Check sheet for the modelled part. Datum: model origin and axes. Units: mm. A direction names the side the tool comes from. Round coordinates to 2 decimals unless told otherwise and drop trailing zeros. Write each loop counter-clockwise with the first axis right and the second up, starting at its lowest first coordinate (ties: lowest second). Pieces come first, ordered by that corner, then holes. Notation, with made-up numbers: (-5.75, 61) - (51.25, 61) arc R22 ccw to (51.25, 71) - close; hole circle Ø11 at (-40, 51). An arc over 180 degrees is marked (long way). Answer as a JSON object with one key per item and string values. Group by question number.
Item 1: Gauge pin test, flat ends, axial feed: P1, Ø8, axis at x = -26.4, y = -15.24, coming from the -Z side; P2, Ø1, axis at y = -29.5, z = 25.5, coming from the +X side; P3, Ø1.5, axis at x = 28, z = 24, coming from the -Y side; P4, Ø3, axis at y = 35, z = 4.5, coming from the -X side. Record the tip position at first contact, or that the pin passes through.
Item 2: Thickness scan on line 1 (Y direction, x = 0, z = 5); line 2 (X direction, y = -11, z = 7.5); line 3 (X direction, y = 13, z = 17.5). Record the ranges inside material, lowest first.
Item 3: Release check for a two-part mould opening along X. For faces 3 (the flat face through (11, 1, 0)), 4 (the cylindrical face through (-27.058, -10.203, 12.878)), 5 (the cylindrical face through (-6.944, -52.886, 17.531)) record: pulls with the +X half, pulls with the -X half, needs draft (parallel to the pull), parting line crosses it, or undercut.
Item 4: Sectioned sample at C-C on z = 10.5. Record the boundary of the cut face in (x, y), plus the area to 3 significant figures.
Item 5: Set-up check for faces 1 (the flat face through (-36, 13, 35.56)), 2 (the flat face through (-1, -8, 25.4)): record each of +Z, -Z, +X, -X, +Y, -Y from which the full face is reachable in a straight line by a thin tool's end or side.
Item 6: Sectioned sample at B-B on y = 0. Record the boundary of the cut face in (x, z).
Item 7: Sectioned sample at D-D on y = 15.24. Record the boundary of the cut face in (x, z), plus the area to 3 significant figures.
Item 8: Sectioned sample at A-A on x = 0. Record the boundary of the cut face in (y, z).
Autodesk Inventor part; units mm, degrees
ref_plane "YZ Plane" through (0, 0, 0) normal (1, 0, 0) x (0, 1, 0)
ref_plane "XZ Plane" through (0, 0, 0) normal (0, 1, 0) x (-1, 0, 0)
ref_plane "XY Plane" through (0, 0, 0) normal (0, 0, 1) x (1, 0, 0)
sketch "Sketch1" plane through (0, 0, 0) normal (0, 0, 1) x (1, 0, 0)
  circle A0 centre (0, 0) radius 53.34
  dimension "d0" = 106.68
extrude "Extrusion1" add sketch "Sketch1" along normal blind 35.56
sketch "Sketch2" plane through (0, 0, 35.56) normal (0, 0, 1) x (1, 0, 0)
  circle A0 centre (0, 0) radius 38.1
  dimension "d3" = 76.2
extrude "Extrusion2" cut sketch "Sketch2" against normal blind 10.16
sketch "Sketch3" plane through (0, 0, 25.4) normal (0, 0, 1) x (1, 0, 0)
  line L0 (-74.676, 0) -> (74.676, 0) construction
  line L1 (0, -74.676) -> (0, 74.676) construction
  circle A0 centre (0, 0) radius 30.48
  circle A1 centre (0, 30.48) radius 5.08
  circle A2 centre (-26.3965, 15.24) radius 5.08
  circle A3 centre (-26.3965, -15.24) radius 5.08
  circle A4 centre (0, -30.48) radius 5.08
  circle A5 centre (26.3965, -15.24) radius 5.08
  circle A6 centre (26.3965, 15.24) radius 5.08
  circle A7 centre (0, 0) radius 5.08
  dimension "d6" = 60.96
  dimension "d7" = 10.16
  dimension "d10" = 360
  dimension "d14" = 10.16
extrude "Extrusion3" cut sketch "Sketch3" against normal through all contours A6 A0 | A0 A6 | A5 A0 | A0 A5 | A1 A0 | A0 A1 | A4 A0 | A0 A4 | A2 A0 | A0 A2 | A3 A0 | A0 A3 | A7
sketch "Sketch4" plane through (0, 0, 0) normal (1, 0, 0) x (0, 1, 0)
  line L0 (-38.1, 25.4) -> (38.1, 25.4)
  line L1 (53.34, 35.56) -> (-53.34, 35.56)
  line L2 (53.34, 0) -> (-53.34, 0)
  line L3 (-5.08, 25.4) -> (-5.08, 0)
  line L4 (-5.08, 0) -> (-25.4, 0)
  line L5 (-25.4, 0) -> (-25.4, 25.4)
  line L6 (-25.4, 25.4) -> (-5.08, 25.4)
  line L7 (5.08, 0) -> (5.08, 25.4)
  line L8 (5.08, 25.4) -> (25.4, 25.4)
  line L9 (25.4, 25.4) -> (25.4, 0)
  line L10 (25.4, 0) -> (5.08, 0)
  line L11 (53.34, 35.56) -> (53.34, 0)
  line L12 (53.34, 0) -> (35.56, 0)
  line L13 (35.56, 0) -> (35.56, 25.4)
  line L14 (35.56, 25.4) -> (38.1, 25.4)
  line L15 (38.1, 25.4) -> (38.1, 35.56)
  line L16 (38.1, 35.56) -> (53.34, 35.56)
  line L17 (-53.34, 0) -> (-53.34, 35.56)
  line L18 (-53.34, 35.56) -> (-38.1, 35.56)
  line L19 (-38.1, 35.56) -> (-38.1, 25.4)
  line L20 (-38.1, 25.4) -> (-35.56, 25.4)
  line L21 (-35.56, 25.4) -> (-35.56, 0)
  line L22 (-35.56, 0) -> (-53.34, 0)
  line L23 (-5.08, 25.4) -> (-5.08, 0)
  line L24 (-5.08, 0) -> (-25.4, 0)
  line L25 (-25.4, 0) -> (-25.4, 25.4)
  line L26 (-25.4, 25.4) -> (-5.08, 25.4)
  line L27 (5.08, 0) -> (5.08, 25.4)
  line L28 (5.08, 25.4) -> (25.4, 25.4)
  line L29 (25.4, 25.4) -> (25.4, 0)
  line L30 (25.4, 0) -> (5.08, 0)
  line L31 (53.34, 35.56) -> (53.34, 0)
  line L32 (53.34, 0) -> (35.56, 0)
  line L33 (35.56, 0) -> (35.56, 25.4)
  line L34 (35.56, 25.4) -> (38.1, 25.4)
  line L35 (38.1, 25.4) -> (38.1, 35.56)
  line L36 (38.1, 35.56) -> (53.34, 35.56)
  line L37 (-53.34, 0) -> (-53.34, 35.56)
  line L38 (-53.34, 35.56) -> (-38.1, 35.56)
  line L39 (-38.1, 35.56) -> (-38.1, 25.4)
  line L40 (-38.1, 25.4) -> (-35.56, 25.4)
  line L41 (-35.56, 25.4) -> (-35.56, 0)
  line L42 (-35.56, 0) -> (-53.34, 0)
  line L43 (-5.08, 25.4) -> (-5.08, 0)
  line L44 (-5.08, 0) -> (-25.4, 0)
  line L45 (-25.4, 0) -> (-25.4, 25.4)
  line L46 (-25.4, 25.4) -> (-5.08, 25.4)
  line L47 (5.08, 0) -> (5.08, 25.4)
  line L48 (5.08, 25.4) -> (25.4, 25.4)
  line L49 (25.4, 25.4) -> (25.4, 0)
  line L50 (25.4, 0) -> (5.08, 0)
  line L51 (53.34, 35.56) -> (53.34, 0)
  line L52 (53.34, 0) -> (35.56, 0)
  line L53 (35.56, 0) -> (35.56, 25.4)
  line L54 (35.56, 25.4) -> (38.1, 25.4)
  line L55 (38.1, 25.4) -> (38.1, 35.56)
  line L56 (38.1, 35.56) -> (53.34, 35.56)
  line L57 (-53.34, 0) -> (-53.34, 35.56)
  line L58 (-53.34, 35.56) -> (-38.1, 35.56)
  line L59 (-38.1, 35.56) -> (-38.1, 25.4)
  line L60 (-38.1, 25.4) -> (-35.56, 25.4)
  line L61 (-35.56, 25.4) -> (-35.56, 0)
  line L62 (-35.56, 0) -> (-53.34, 0)
  line L63 (53.34, 35.56) -> (-53.34, 35.56)
  line L64 (53.34, 0) -> (-53.34, 0)
  line L65 (53.34, 0) -> (-53.34, 0) construction
  line L66 (12.7, 0) -> (12.7, 35.56) construction
  line L67 (-12.7, 0) -> (-12.7, 35.56) construction
  line L68 (0, -7.112) -> (0, 42.672)
  line L69 (48.26, 0) -> (12.7, 0)
  line L70 (12.7, 0) -> (12.7, 10.16)
  line L71 (12.7, 10.16) -> (48.26, 10.16)
  line L72 (48.26, 10.16) -> (48.26, 0)
  point P0 (0, 0)
  point P1 (0, 35.56)
  point P2 (0, 25.4)
  dimension "d15" = 25.4
  dimension "d16" = 10.16
  dimension "d17" = 5.08
  dimension "d18" = 7.62
revolve "Revolution1" cut sketch "Sketch4" angle 360 about axis through (0, 0, -10) along (0, 0, 1) contours L1 L15 L0 L68
equation "\"BendRadius\" = Thickness"
equation "\"BendReliefWidth\" = Thickness"
equation "\"BendReliefDepth\" = 0.5 * Thickness"
equation "\"CornerReliefSize\" = 4 * Thickness"
equation "\"MinimumRemnant\" = 2 * Thickness"
equation "\"TransitionRadius\" = BendRadius"
equation "\"JacobiRadiusSize\" = BendRadius"
equation "\"GapSize\" = Thickness"
properties part number "valve" material "Brass, Soft Yellow"
Completed:
{
 "1": {"P1": "through", "P2": "x = 44.77", "P3": "y = -45.85", "P4": "x = -41.51"},
 "2": {"line 1": "-53.34 to -35.56, -25.4 to -5.08, 5.08 to 25.4, 35.56 to 53.34", "line 2": "-52.19 to -29.19, -23.6 to 23.6, 29.19 to 52.19", "line 3": "-51.73 to -30.96, -21.84 to 21.84, 30.96 to 51.73"},
 "3": {"face 3": "needs draft", "face 4": "undercut", "face 5": "parting line crosses it"},
 "4": {"outline": "circle Ø106.68 at (0, 0); hole circle Ø10.16 at (-26.4, -15.24); hole circle Ø10.16 at (-26.4, 15.24); hole circle Ø10.16 at (0, -30.48); hole circle Ø10.16 at (0, 0); hole circle Ø10.16 at (0, 30.48); hole circle Ø10.16 at (26.4, -15.24); hole circle Ø10.16 at (26.4, 15.24)", "area": "8,370 mm²"},
 "5": {"face 1": "+Z, +X, -X, +Y, -Y", "face 2": "+Z"},
 "6": {"outline": "(-53.34, 0) - (-5.08, 0) - (-5.08, 25.4) - (-38.1, 25.4) - (-38.1, 35.56) - (-53.34, 35.56) - close; (5.08, 0) - (53.34, 0) - (53.34, 35.56) - (38.1, 35.56) - (38.1, 25.4) - (5.08, 25.4) - close"},
 "7": {"outline": "(-51.12, 0) - (-31.48, 0) - (-31.48, 25.4) - (-34.92, 25.4) - (-34.92, 35.56) - (-51.12, 35.56) - close; (-21.32, 0) - (21.32, 0) - (21.32, 25.4) - (-21.32, 25.4) - close; (31.48, 0) - (51.12, 0) - (51.12, 35.56) - (34.92, 35.56) - (34.92, 25.4) - (31.48, 25.4) - close", "area": "2,410 mm²"},
 "8": {"outline": "(-53.34, 0) - (-35.56, 0) - (-35.56, 25.4) - (-38.1, 25.4) - (-38.1, 35.56) - (-53.34, 35.56) - close; (-25.4, 0) - (-5.08, 0) - (-5.08, 25.4) - (-25.4, 25.4) - close; (5.08, 0) - (25.4, 0) - (25.4, 25.4) - (5.08, 25.4) - close; (35.56, 0) - (53.34, 0) - (53.34, 35.56) - (38.1, 35.56) - (38.1, 25.4) - (35.56, 25.4) - close"}
}
